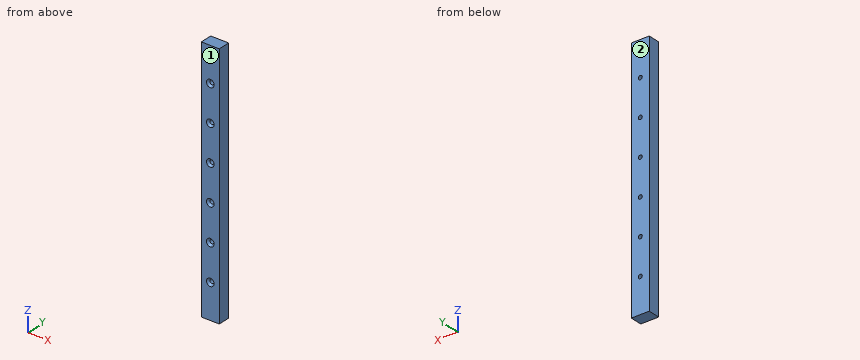
```python
from build123d import *

# Parameters (mm, degrees)
SKETCH1_W                                         = 38.1
SKETCH1_H                                         = 25.4
BOSS_EXTRUDE1_DEPTH                               = 527.05
CSK_FOR_5_16_FLAT_HEAD_MACHINE_SCREW1_D           = 8.4328
CSK_FOR_5_16_FLAT_HEAD_MACHINE_SCREW1_CSINK_D     = 16.129
CSK_FOR_5_16_FLAT_HEAD_MACHINE_SCREW1_CSINK_ANGLE = 82


with BuildPart() as part:
    # Sketch1 → Boss-Extrude1 (new body)
    with BuildSketch(Plane.XY):
        with Locations((-3.175, 0)):
            Rectangle(SKETCH1_W, SKETCH1_H)
    extrude(amount=BOSS_EXTRUDE1_DEPTH)

    # CSK for 5/16 Flat Head Machine Screw1 (through all)
    with Locations(Plane(origin=(0, -12.7, 0), x_dir=(-1, 0, 0), z_dir=(0, -1, 0))):
        with Locations((3.175, -454.025), (3.175, -377.825), (3.175, -301.625), (3.175, -225.425), (3.175, -149.225), (3.175, -73.025)):
            CounterSinkHole(CSK_FOR_5_16_FLAT_HEAD_MACHINE_SCREW1_D / 2, CSK_FOR_5_16_FLAT_HEAD_MACHINE_SCREW1_CSINK_D / 2, counter_sink_angle=CSK_FOR_5_16_FLAT_HEAD_MACHINE_SCREW1_CSINK_ANGLE)


solid = part.part
```
Geometry check sheet. Reference: the model listing, model coordinates, mm. Face numbers are marked on the shaded views. Coordinates: 2 decimals unless noted, no trailing zeros. Loops run counter-clockwise (first coordinate to the right, second up) from the corner with the lowest first, then second, coordinate; pieces in that order, holes last. Notation, with made-up numbers: (13.25, 27) - (66.25, 27) arc R14 cw to (66.25, 39) - close; hole circle Ø6 at (44.25, 44). An arc over 180 degrees is marked (long way). One line per item, written item: value. Start each with the question number.
(1) Cross-section at A-A on y = 4. Enter the section's corners in (x, z) (3 decimals).
(2) Material ranges on line 1 (X direction, y = -2.5, z = 451.5) (3 decimals); line 2 (X direction, y = 5.75, z = 228.5) (3 decimals), recorded low to high. Write a range as [from, to].
(3) Mould release check, pull along Y, two halves, no side actions. Record for the marked faces 1 and 2: released by +Y, released by -Y, zero draft, split by the parting line, or undercut.
(4) Depth check by flat-ended pin: P1, Ø13.5, axis at x = -3.175, z = 225.425, coming from the -Y side; P2, Ø9.5, axis at x = -3.175, z = 377.825, coming from the -Y side. Enter the tip coordinate at first touch or a pass-through.
Results below:
1. outline: (-22.225, 0) - (15.875, 0) - (15.875, 527.05) - (-22.225, 527.05) - close; hole circle Ø8.433 at (-3.175, 73.025); hole circle Ø8.433 at (-3.175, 149.225); hole circle Ø8.433 at (-3.175, 225.425); hole circle Ø8.433 at (-3.175, 301.625); hole circle Ø8.433 at (-3.175, 377.825); hole circle Ø8.433 at (-3.175, 454.025)
2. line 1: x = [-22.225, -6.552], [0.202, 15.875]
2. line 2: x = [-22.225, -6.06], [-0.29, 15.875]
3. face 1: released by -Y
3. face 2: released by +Y
4. P1: stops at y = -11.19
4. P2: stops at y = -8.89
